from build123d import *

# Parameters (mm, degrees)
F0_W     = 30
F0_H     = 10
F1_DEPTH = 25
F2_R     = 1.25
F3_DEPTH = 2
F4_R     = 0.5
F5_DEPTH = 10


with BuildPart() as f1:
    # F0 (on Front) → F1 (new body)
    with BuildSketch(Plane.XZ):
        with Locations((-31.001214, 5)):
            Rectangle(F0_W, F0_H)
    extrude(amount=-F1_DEPTH)

    # F2 (on face) → F3 (join)
    with BuildSketch(Plane.XZ):
        with Locations((-22.001214, 5)):
            Circle(F2_R)
    extrude(amount=F3_DEPTH)

    # F4 (on face) → F5 (join)
    with BuildSketch(Plane.XZ):
        with Locations((-43.001214, 7)):
            Circle(F4_R)
    extrude(amount=F5_DEPTH)


solid = f1.part
Input: part model. Units: mm. Frame: model coordinates. A direction names the side the tool comes from. Round coordinates to 2 decimals unless told otherwise and drop trailing zeros. Order: outer loops, then holes, each group sorted by start corner. A loop starts at its lowest first (then second) coordinate and runs counter-clockwise, first axis right, second up. Notation, with made-up numbers: (-12.5, 14) - (23.5, 14) arc R12 ccw to (23.5, 24) - close; hole circle Ø2 at (6, -17). An arc over 180 degrees is marked (long way). Answer as a JSON object with one key per item and string values. Group by question number.
(1) Reachability of faces 1 (the face through (-43.11, -4.93, 6.51)), 2 (the face through (-22, -2, 5)) from +Z, -Z, +X, -X, +Y, -Y: full face, straight path, thin tool, end or side. Return the list, or none.
(2) Cut plane A-A (z = 5). Return loops of the section in (x, y), then the cut area to 3 significant figures.
(3) Cut plane C-C (x = -33.5). Return loops of the section in (y, z).
(4) Cut plane D-D (z = 7). Return loops of the section in (x, y).
(5) Material intervals for probe 1 along Y at (x, z) = (-39, 4.75), sorted ascending. Write a range as from..to.
(6) Cut plane B-B (y = -0.5). Return loops of the section in (x, z).
(7) Pin query (flat end, axial travel): P1, Ø3, axis at y = -2.5, z = 6, coming from the -X side; P2, Ø1.2, axis at x = -21.5, z = 5, coming from the -Y side; P3, Ø3, axis at x = -24.5, z = 3, coming from the -Y side. Return the tip coordinate at first contact, or that it passes through.
Here are the results:
{
 "1": {"face 1": "-Y", "face 2": "+Z, -Z, +X, -X, -Y"},
 "2": {"outline": "(-46, 0) - (-23.25, 0) - (-23.25, -2) - (-20.75, -2) - (-20.75, 0) - (-16, 0) - (-16, 25) - (-46, 25) - close", "area": "755 mm^2"},
 "3": {"outline": "(0, 0) - (25, 0) - (25, 10) - (0, 10) - close"},
 "4": {"outline": "(-46, 0) - (-43.5, 0) - (-43.5, -10) - (-42.5, -10) - (-42.5, 0) - (-16, 0) - (-16, 25) - (-46, 25) - close"},
 "5": {"probe 1": "y = 0..25"},
 "6": {"outline": "circle Ø1 at (-43, 7); circle Ø2.5 at (-22, 5)"},
 "7": {"P1": "stops at x = -43.5", "P2": "stops at y = -2", "P3": "stops at y = 0"}
}
